Design review of the part shown in the three views and the two pictorial views. Dimensions are in mm from the part's minimum x, y and z. Round coordinates to 2 decimals unless told otherwise and drop trailing zeros. Order: outer loops, then holes, each group sorted by start corner. A loop starts at its lowest first (then second) coordinate and runs counter-clockwise, first axis right, second up. Notation, with made-up numbers: (1.25, 20) - (58.25, 20) arc R31 ccw to (58.25, 53) - close; hole circle Ø1 at (64, -6.75). An arc over 180 degrees is marked (long way). Use CSV: the item, a comma, the result in double quotes.
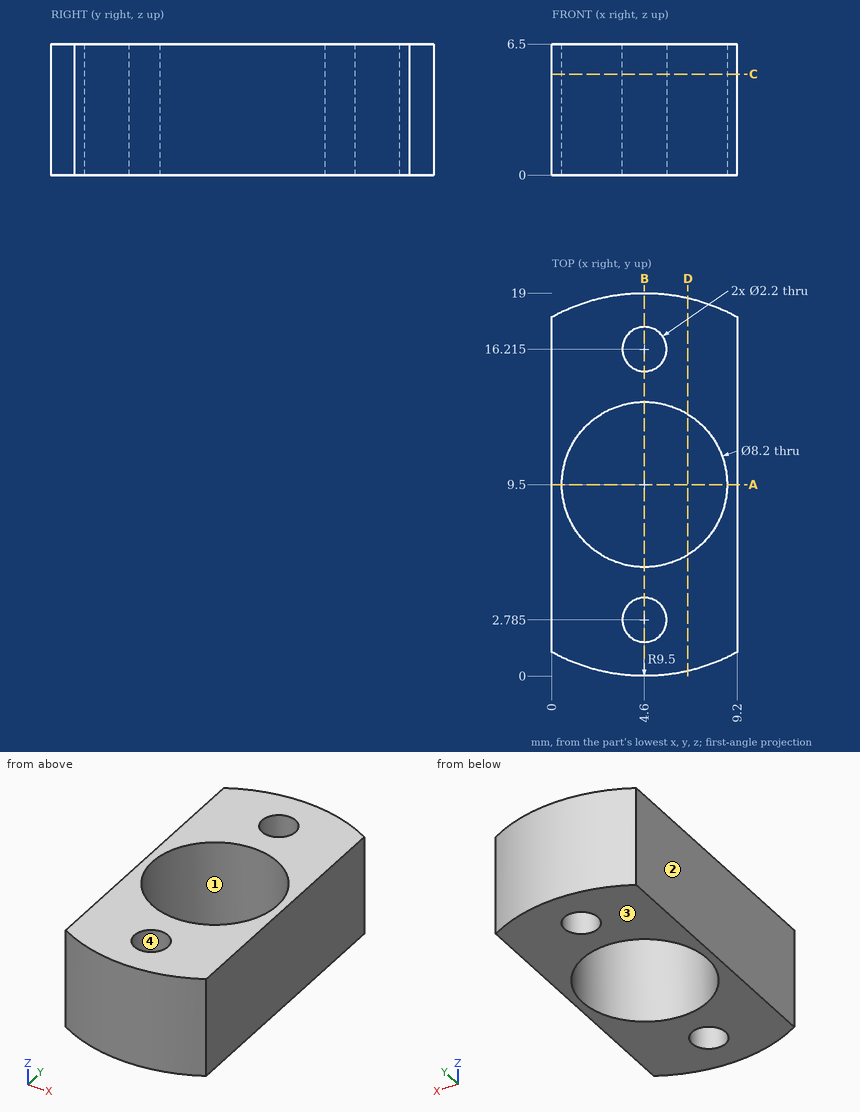
1) We need section C-C (z = 5). Give the boundary of the cut face in (x, y) (3 decimals), then the cut area to 3 significant figures.
Data:
outline,"(0, 1.188) arc R9.5 ccw to (9.2, 1.188) - (9.2, 17.812) arc R9.5 ccw to (0, 17.812) - close; hole circle Ø8.2 at (4.6, 9.5); hole circle Ø2.2 at (4.6, 2.785); hole circle Ø2.2 at (4.6, 16.215)"
area,"107 mm2"
2) To check wall thickness, follow L1, parallel to Y at x = 5, z = 4; L2, parallel to Y at x = 2.75, z = 1.25; L3, parallel to Y at x = 7.5, z = 3.75. State the ranges of each line that lie inside material, in increasing order. Write a range as from..to.
Data:
L1,"y = 0.01..1.76, 3.81..5.42, 13.58..15.19, 17.24..18.99"
L2,"y = 0.18..5.84, 13.16..18.82"
L3,"y = 0.45..6.6, 12.4..18.55"
3) The part is to be moulded in two halves that separate along X. For the marked faces 1, 2, 3 and 4, say which applies: +X half, -X half, draft (parallel to the pull), parting line (faces both ways), or undercut.
Data:
face 1,"undercut"
face 2,"-X half"
face 3,"draft"
face 4,"undercut"
4) We need section A-A (y = 9.5). Give the boundary of the cut face in (x, z).
Data:
outline,"(0, 0) - (0.5, 0) - (0.5, 6.5) - (0, 6.5) - close; (8.7, 0) - (9.2, 0) - (9.2, 6.5) - (8.7, 6.5) - close"
5) We need section D-D (x = 6.75). Give the boundary of the cut face in (y, z).
Data:
outline,"(0.25, 0) - (6.01, 0) - (6.01, 6.5) - (0.25, 6.5) - close; (12.99, 0) - (18.75, 0) - (18.75, 6.5) - (12.99, 6.5) - close"
6) We need section B-B (x = 4.6). Give the boundary of the cut face in (y, z) (3 decimals).
Data:
outline,"(0, 0) - (1.685, 0) - (1.685, 6.5) - (0, 6.5) - close; (3.885, 0) - (5.4, 0) - (5.4, 6.5) - (3.885, 6.5) - close; (13.6, 0) - (15.115, 0) - (15.115, 6.5) - (13.6, 6.5) - close; (17.315, 0) - (19, 0) - (19, 6.5) - (17.315, 6.5) - close"
